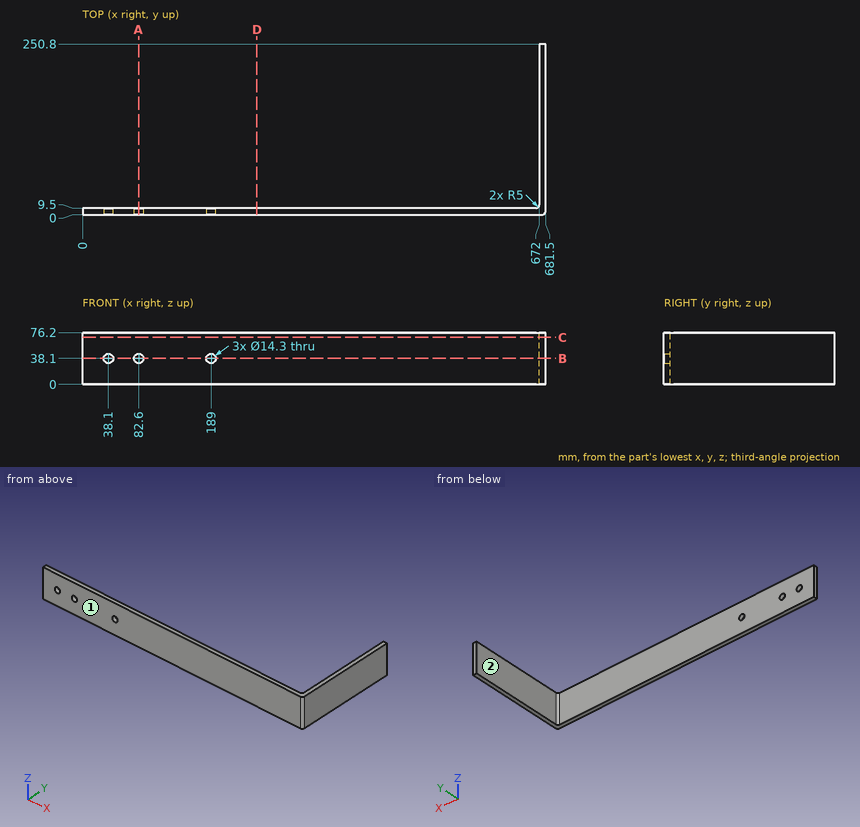
Verification items for this drawing (mm, ordinates from the low corner). A direction names the side the tool comes from. Give positions to 0.01 mm unless a question says otherwise; leave off trailing zeros. Loops run counter-clockwise (first coordinate to the right, second up) from the corner with the lowest first, then second, coordinate; pieces in that order, holes last.
(1) Section check C-C on z = 69. Record the cut outline in (x, y).
From the geometry:
outline: (0, 0) - (676.5, 0) arc R5 ccw to (681.5, 5) - (681.5, 250.8) - (672, 250.8) - (672, 14.5) arc R5 cw to (667, 9.5) - (0, 9.5) - close
(2) Section check D-D on x = 256.5. Record the cut outline in (y, z), then the cut area to 3 significant figures.
From the geometry:
outline: (0, 0) - (9.5, 0) - (9.5, 76.2) - (0, 76.2) - close
area: 724 mm2
(3) Depth check by flat-ended pin: pin 1 Ø5 at (x, z) = (233.5, 65.5) entering from +Y; pin 2 Ø1 at (y, z) = (80.5, 52) entering from -X; pin 3 Ø8.5 at (x, z) = (38.1, 38.1) entering from +Y. Enter the tip coordinate at first touch or a pass-through.
From the geometry:
pin 1: stops at y = 9.5
pin 2: stops at x = 672
pin 3: passes through
(4) Set-up check for the marked faces 1 and 2: record each of +Z, -Z, +X, -X, +Y, -Y from which the full face is reachable in a straight line by a thin tool's end or side.
From the geometry:
face 1: +Z, -Z, +X, -X, -Y
face 2: +Z, -Z, -X, +Y
(5) Section check B-B on z = 38.1. Record the cut outline in (x, y), then the cut area to 3 significant figures.
From the geometry:
outline: (0, 0) - (30.95, 0) - (30.95, 9.5) - (0, 9.5) - close; (45.25, 0) - (75.45, 0) - (75.45, 9.5) - (45.25, 9.5) - close; (89.75, 0) - (181.85, 0) - (181.85, 9.5) - (89.75, 9.5) - close; (196.15, 0) - (676.5, 0) arc R5 ccw to (681.5, 5) - (681.5, 250.8) - (672, 250.8) - (672, 14.5) arc R5 cw to (667, 9.5) - (196.15, 9.5) - close
area: 8,360 mm2
(6) Section check A-A on x = 82.6. Record the cut outline in (y, z), then the cut area to 3 significant figures.
From the geometry:
outline: (0, 0) - (9.5, 0) - (9.5, 30.95) - (0, 30.95) - close; (0, 45.25) - (9.5, 45.25) - (9.5, 76.2) - (0, 76.2) - close
area: 588 mm2
(7) Thickness scan on L1, parallel to Z at x = 38.1, y = 5.5; L2, parallel to X at y = 194.5, z = 43; L3, parallel to Y at x = 422.5, z = 64.5. Record the ranges inside material, lowest first.
From the geometry:
L1: z = 0 to 30.95, 45.25 to 76.2
L2: x = 672 to 681.5
L3: y = 0 to 9.5
